```python
from build123d import *

# Parameters (mm, degrees)
EXTRUDE_4_DEPTH     = 10
EXTRUDE_8_DEPTH     = 20
SKETCH_16_W         = 8
SKETCH_16_H         = 40
SKETCH_19_W         = 8
SKETCH_19_H         = 40
SKETCH_21_R         = 16
EXTRUDE_13_DEPTH    = 8
SKETCH_22_R         = 16
EXTRUDE_14_DEPTH    = 8
SKETCH_23_W         = 7.590296008
SKETCH_23_H         = 50
CUT_EXTRUDE_2_DEPTH = 314.490031739
EXTRUDE_15_DEPTH    = 40
SKETCH_29_W         = 8
SKETCH_29_H         = 20
EXTRUDE_19_DEPTH    = 40
SKETCH_33_R         = 10
EXTRUDE_22_DEPTH    = 10
SKETCH_34_R         = 10
EXTRUDE_23_DEPTH    = 10


with BuildPart() as part:
    # Sketch 3D_1 → Extrude 4 (new, symmetric)
    with BuildSketch(Plane(origin=(-74, 270, 0), x_dir=(0.9909924304103234, 0, 0.13391789600139506), z_dir=(0, -1, 0))):
        with BuildLine():
            Line((0, 0), (2.67835792, 19.819848608))
            Line((2.67835792, 19.819848608), (10.606297363, 18.74850544))
            Line((10.606297363, 18.74850544), (7.927939443, -1.071343168))
            ThreePointArc((7.927939443, -1.071343168), (64.494858714, -75.315424711), (138.738940257, -18.74850544))
            Line((138.738940257, -18.74850544), (141.417298177, 1.071343168))
            Line((141.417298177, 1.071343168), (149.345237621, 0))
            Line((149.345237621, 0), (146.666879701, -19.819848608))
            ThreePointArc((146.666879701, -19.819848608), (63.423515546, -83.243364154), (0, 0))
        make_face()
    extrude(amount=EXTRUDE_4_DEPTH, both=True)



with BuildPart() as body_2:
    # Sketch 3D_2 → Extrude 8 (new body)
    with BuildSketch(Plane(origin=(-46, 50, 0), x_dir=(0.9771763639228009, 0, 0.2124296443310437), z_dir=(0, 1, 0))):
        with BuildLine():
            Line((0, 0), (4.248592887, -19.543527278))
            Line((4.248592887, -19.543527278), (12.066003798, -17.844090124))
            Line((12.066003798, -17.844090124), (7.817410911, 1.699437155))
            Line((7.817410911, 1.699437155), (3.568818025, 21.242964433))
            ThreePointArc((3.568818025, 21.242964433), (32.629193369, 66.447992747), (77.834221683, 37.387617402))
            Line((77.834221683, 37.387617402), (82.08281457, 17.844090124))
            Line((82.08281457, 17.844090124), (86.331407456, -1.699437155))
            Line((86.331407456, -1.699437155), (94.148818368, 0))
            Line((94.148818368, 0), (89.900225481, 19.543527278))
            Line((89.900225481, 19.543527278), (85.651632594, 39.087054557))
            ThreePointArc((85.651632594, 39.087054557), (30.929756215, 74.265403658), (-4.248592887, 19.543527278))
            Line((-4.248592887, 19.543527278), (0, 0))
        make_face()
    extrude(amount=EXTRUDE_8_DEPTH)


with BuildPart() as part_1:
    add(part.part)

    add(body_2.part)  # Sweep 5 merges body 2
    # Sweep 5: sweep along a path in Sketch 18
    with BuildLine(Plane.XY.offset(20)) as sweep_5_path:
        Line((-46, 0), (-46, 50))
        Line((-46, 50), (-46, 70))
        Line((-46, 70), (-74, 260))
        Line((-74, 260), (-74, 280))
    # Sketch 16 → Sweep 5 (sweep)
    with BuildSketch(Plane(origin=(0, 0, 0), x_dir=(1, 0, 0), z_dir=(0, 1, 0))):
        with Locations((-42, 0)):
            Rectangle(SKETCH_16_W, SKETCH_16_H)
    sweep(path=sweep_5_path.line, transition=Transition.RIGHT)

    # Sweep 6: sweep along a path in Sketch 20
    with BuildLine(Plane.XY.offset(20)) as sweep_6_path:
        Line((46, 0), (46, 50))
        Line((46, 50), (46, 70))
        Line((46, 70), (74, 260))
        Line((74, 260), (74, 280))
    # Sketch 19 → Sweep 6 (sweep)
    with BuildSketch(Plane(origin=(0, 0, 0), x_dir=(1, 0, 0), z_dir=(0, 1, 0))):
        with Locations((42, 0)):
            Rectangle(SKETCH_19_W, SKETCH_19_H)
    sweep(path=sweep_6_path.line, transition=Transition.RIGHT)

    # Sketch 21 → Extrude 13 (add)
    with BuildSketch(Plane(origin=(46, 0, 0), x_dir=(0, 0, -1), z_dir=(1, 0, 0))):
        Circle(SKETCH_21_R)
    extrude(amount=-EXTRUDE_13_DEPTH)

    # Sketch 22 → Extrude 14 (add)
    with BuildSketch(Plane.ZY.offset(46)):
        Circle(SKETCH_22_R)
    extrude(amount=-EXTRUDE_14_DEPTH)

    # Sketch 23 → Cut-Extrude 2 (cut, through all)
    with BuildSketch(Plane.ZY.offset(46)):
        with Locations((19.795148004, 25)):
            Rectangle(SKETCH_23_W, SKETCH_23_H)
    extrude(amount=-CUT_EXTRUDE_2_DEPTH, mode=Mode.SUBTRACT)

    # Sketch 25 → Extrude 15 (add)
    with BuildSketch(Plane.XZ.offset(-260)):
        with BuildLine():
            Line((71.246052522, 20), (75.3923073, 20))
            ThreePointArc((75.3923073, 20), (0, -78), (-75.3923073, 20))
            Line((-75.3923073, 20), (-71.246052522, 20))
            ThreePointArc((-71.246052522, 20), (0, -74), (71.246052522, 20))
        make_face()
    extrude(amount=-EXTRUDE_15_DEPTH)

    # Sketch 29 → Extrude 19 (add)
    with BuildSketch(Plane.XY.offset(20)):
        with Locations((-50, 60)):
            Rectangle(SKETCH_29_W, SKETCH_29_H)
        with Locations((50, 60)):
            Rectangle(SKETCH_29_W, SKETCH_29_H)
    extrude(amount=-EXTRUDE_19_DEPTH)

    # Sketch 33 → Extrude 22 (add)
    with BuildSketch(Plane.ZY.offset(54)):
        with Locations((10, 60)):
            Circle(SKETCH_33_R)
    extrude(amount=EXTRUDE_22_DEPTH)

    # Sketch 34 → Extrude 23 (add)
    with BuildSketch(Plane(origin=(54, 0, 0), x_dir=(0, 0, -1), z_dir=(1, 0, 0))):
        with Locations(Location((-10, 60, 0), (0, 0, 180))):
            Circle(SKETCH_34_R)
    extrude(amount=EXTRUDE_23_DEPTH)


solid = part_1.part
```
Input: part model. Units: mm. Frame: model coordinates. A direction names the side the tool comes from. Give positions to 0.01 mm unless a question says otherwise; leave off trailing zeros. Write each loop counter-clockwise with the first axis right and the second up, starting at its lowest first coordinate (ties: lowest second). Pieces come first, ordered by that corner, then holes. Notation, with made-up numbers: (66, 32) - (91, 32) arc R25 cw to (91, 47) - close; hole circle Ø10 at (79, 76.25). An arc over 180 degrees is marked (long way). Write item = value, one per line. Start each with the question number.
1. Section query C-C, the plane y = 157. Output: boundary loops of the cut face in (x, z).
2. Access query for faces 1 (the flat face through (-2.8, 70, -58.3)), 2 (the flat face through (49, 50, 0)), 3 (the flat face through (56, 172, -20)), 4 (the flat face through (-42, 25, -20)), 5 (the flat face through (46, 17, -2)). Directions: +Z, -Z, +X, -X, +Y, -Y. A direction counts if a zero-diameter tool reaches every point of the face in a straight line with its end or side. Return the directions, or none.
3. Ray query, L1, parallel to X at y = 286.5, z = 0; L2, parallel to X at y = 68, z = -15; L3, parallel to Z at x = 0, y = 285.75. Return the intervals inside material, ascending.
4. Section query D-D, the plane z = -50. Output: boundary loops of the cut face in (x, y), then the cut area to 3 significant figures.
5. Mould query, pull axis X, two halves, no side actions, for faces 6 (the flat face through (-54, 60, -8)), 7 (the flat face through (-52.196, 166.916, 0.28)), 8 (the flat face through (-50, 60, -20)). Classes: released by +X, released by -X, zero draft, split by the parting line, or undercut.
6. Section query B-B, the plane x = 57. Output: boundary loops of the cut face in (y, z), then the cut area to 3 significant figures.
7. Section query A-A, the plane x = 0. Output: boundary loops of the cut face in (y, z).
8. First-contact query: pin 1 Ø3 at (y, z) = (57.5, 15) entering from +X; pin 2 Ø2.5 at (x, y) = (40, 18) entering from -Z; pin 3 Ø16 at (y, z) = (62.5, 14) entering from -X; pin 4 Ø6 at (x, y) = (-55, 97.5) entering from +Z. Flat tips, straight axial feed; report the tip coordinate or a pass-through.
Check sheet entries:
q1.outline = (-58.82, -20) - (-50.73, -20) - (-50.73, 20) - (-58.82, 20) - close; (50.73, -20) - (58.82, -20) - (58.82, 20) - (50.73, 20) - close
q2.face_1 = -Z, +X, -X, +Y
q2.face_2 = +Z, +X, -Y
q2.face_3 = -Z, +X, -X
q2.face_4 = -Z, +X, -X, -Y
q2.face_5 = +Z, -Z, +X, -Y
q3.L1 = -78 to -74, 74 to 78
q3.L2 = -54 to -38, 38 to 54
q3.L3 = -78 to -74
q4.outline = (-59.87, 260) - (-43.08, 260) - (-43.08, 280) - (-54.55, 280) - (-54.55, 300) - (-59.87, 300) - close; (-34.87, 50) - (-23.32, 50) - (-23.32, 70) - (-34.87, 70) - close; (23.32, 50) - (34.87, 50) - (34.87, 70) - (23.32, 70) - close; (43.08, 260) - (59.87, 260) - (59.87, 300) - (54.55, 300) - (54.55, 280) - (43.08, 280) - close
q4.area = 1,350 mm2
q5.face_6 = released by -X
q5.face_7 = undercut
q5.face_8 = zero draft
q6.outline = circle Ø20 at (60, 10); (144.64, -20) - (199.51, -20) - (199.51, 20) - (144.64, 20) - close; (260, -53.24) - (300, -53.24) - (300, -47.19) - (280, -47.19) - (280, -33.27) - (260, -33.27) - close
q6.area = 3,030 mm2
q7.outline = (50, -66) - (70, -66) - (70, -58) - (50, -58) - close; (260, -78) - (300, -78) - (300, -74) - (280, -74) - (280, -66) - (260, -66) - close
q8.pin_1 = 64
q8.pin_2 = -20
q8.pin_3 = -64
q8.pin_4 = through
